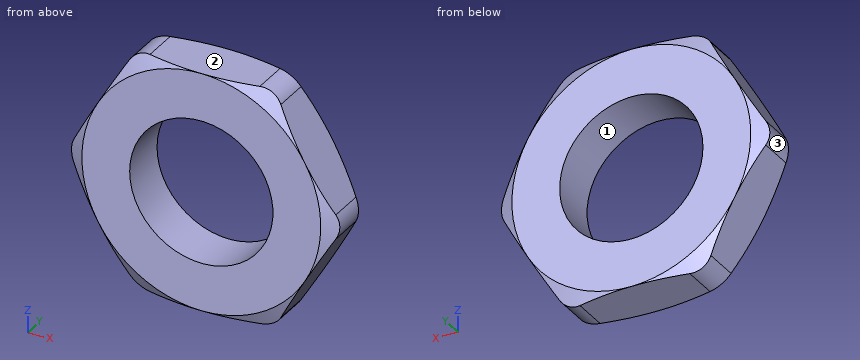
from build123d import *

# Parameters (mm, degrees)
BOSS_EXTRUDE1_DEPTH   = 2
M7X1_0_TAPPED_HOLE1_D = 6
FILLET1_R             = 1.016


with BuildPart() as part:
    # Sketch1 → Boss-Extrude1 (new body)
    with BuildSketch(Plane(origin=(0, 0, 0), x_dir=(1, 0, 0), z_dir=(0, 1, 0))):
        Polygon((-2.886751346, 5), (-5.773502692, 0), (-2.886751346, -5), (2.886751346, -5), (5.773502692, 0), (2.886751346, 5), align=None)
    extrude(amount=BOSS_EXTRUDE1_DEPTH)

    # M7x1.0 Tapped Hole1 (through all)
    with Locations(Plane(origin=(0, 2, 0), x_dir=(1, 0, 0), z_dir=(0, 1, 0))):
        with Locations((0, 0)):
            Hole(M7X1_0_TAPPED_HOLE1_D / 2)

    # Sketch4 → Cut-Revolve1 (revolve, cut)
    with BuildSketch(Plane.XY, mode=Mode.PRIVATE) as cut_revolve1_sk:
        Polygon((5.773502692, 1.6), (5, 2), (5.773502692, 2), align=None)
        Polygon((5.773502692, 0.4), (5.773502692, 0), (5, 0), align=None)
    revolve(cut_revolve1_sk.sketch.rotate(Axis((0, 0, 0), (0, 1, 0)), 270), axis=Axis((0, 0, 0), (0, 1, 0)), mode=Mode.SUBTRACT)

    # Fillet1
    fillet1_edges = [part.edges().sort_by_distance(p)[0] for p in [
        (2.886751346, 1, 5),
        (-2.886751346, 1, 5),
        (-5.773502692, 1, 0),
        (-2.886751346, 1, -5),
        (2.886751346, 1, -5),
        (5.773502692, 1, 0),
    ]]
    fillet(fillet1_edges, radius=FILLET1_R)


solid = part.part
The listing builds one solid part. Answer for the finished solid, in the listing's coordinates (mm). Face numbers are marked on the shaded views. Round coordinates to 2 decimals unless told otherwise and drop trailing zeros. Order: outer loops, then holes, each group sorted by start corner. A loop starts at its lowest first (then second) coordinate and runs counter-clockwise, first axis right, second up. Notation, with made-up numbers: (36.25, 59) -> (92.25, 59) arc R13 cw to (92.25, 70) -> close; hole circle Ø8 at (-22, 66.25). An arc over 180 degrees is marked (long way). Write each question's results on one line, items separated by ' | '. Start each with the question number.
Q1. Straight lines are drawn through the part: probe 1 along Z at (x, y) = (0.5, 0.25); probe 2 along Z at (x, y) = (-0.75, 1.25); probe 3 along X at (y, z) = (0.15, -2.75). For each, find the intervals that lie inside material, in ascending order. Write a range as from..to.
Q2. Find section A-A (z = 0). Determine the outline of the cut face in (x, y), then the cut area to 3 significant figures.
Q3. Find section B-B (y = 0.55). Determine the outline of the cut face in (x, z).
Q4. The mould has two halves that part along X. Classify the marked faces 1, 2 and 3: pulls with the +X half, pulls with the -X half, needs draft (parallel to the pull), parting line crosses it, or undercut.
Worked answers:
1) probe 1: z = -5..-2.96, 2.96..5 | probe 2: z = -5..-2.9, 2.9..5 | probe 3: x = -4.19..-1.2, 1.2..4.19
2) outline: (-5.62, 0.32) -> (-5, 0) -> (-3, 0) -> (-3, 2) -> (-5, 2) -> (-5.62, 1.68) -> close; (3, 0) -> (5, 0) -> (5.62, 0.32) -> (5.62, 1.68) -> (5, 2) -> (3, 2) -> close | area: 10.1 mm2
3) outline: (-5.48, -0.51) -> (-3.18, -4.49) arc R1.02 ccw to (-2.3, -5) -> (2.3, -5) arc R1.02 ccw to (3.18, -4.49) -> (5.48, -0.51) arc R1.02 ccw to (5.48, 0.51) -> (3.18, 4.49) arc R1.02 ccw to (2.3, 5) -> (-2.3, 5) arc R1.02 ccw to (-3.18, 4.49) -> (-5.48, 0.51) arc R1.02 ccw to start; hole circle Ø6 at (0, 0)
4) face 1: undercut | face 2: needs draft | face 3: pulls with the -X half
